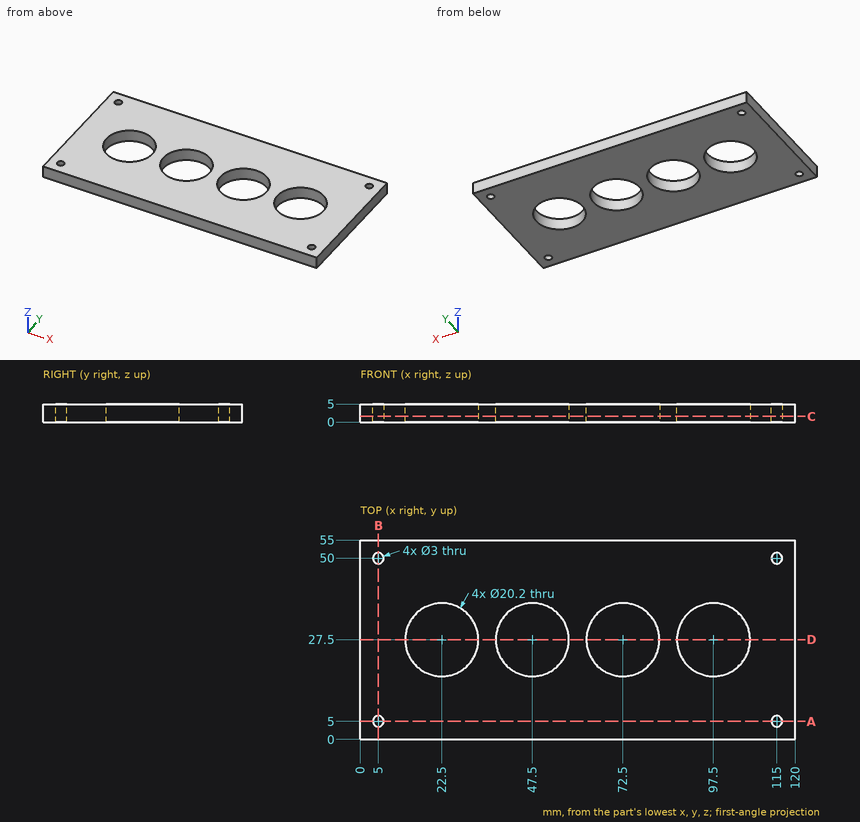
Print and shaded views of the part. All mm, measured from the part's lowest x, y and z. Give positions to 0.01 mm unless a question says otherwise; leave off trailing zeros. Write each loop counter-clockwise with the first axis right and the second up, starting at its lowest first coordinate (ties: lowest second). Pieces come first, ordered by that corner, then holes. Notation, with made-up numbers: (-32.75, 86.25) -> (5.25, 86.25) arc R26 cw to (5.25, 106.25) -> close; hole circle Ø11 at (-23.75, 88). An arc over 180 degrees is marked (long way). Write item = value, one per line.
(1) Slice it at A-A, the plane y = 5. Give the cut face in (x, z), then the cut area to 3 significant figures.
Determined:
outline = (0, 0) -> (3.5, 0) -> (3.5, 5) -> (0, 5) -> close; (6.5, 0) -> (113.5, 0) -> (113.5, 5) -> (6.5, 5) -> close; (116.5, 0) -> (120, 0) -> (120, 5) -> (116.5, 5) -> close
area = 570 mm2
(2) Slice it at C-C, the plane z = 1.6. Give the number of separate pieces and of enclosed holes in the cut face, then the cut area to 3 significant figures.
Determined:
separate_pieces = 1
enclosed_holes = 8
area = 5,290 mm2
(3) Probe line 1 along X through (y, z) = (22.5, 3); line 2 along X through (y, z) = (19, 2.05); line 3 along Y through (x, z) = (72.5, 2.7). List the from-to ranges inside material, lowest first.
Determined:
line_1 = 0 to 13.72, 31.28 to 38.72, 56.28 to 63.72, 81.28 to 88.72, 106.28 to 120
line_2 = 0 to 17.04, 27.96 to 42.04, 52.96 to 67.04, 77.96 to 92.04, 102.96 to 120
line_3 = 0 to 17.4, 37.6 to 55
(4) Slice it at B-B, the plane x = 5. Give the cut face in (y, z), then the cut area to 3 significant figures.
Determined:
outline = (0, 0) -> (3.5, 0) -> (3.5, 5) -> (0, 5) -> close; (6.5, 0) -> (48.5, 0) -> (48.5, 5) -> (6.5, 5) -> close; (51.5, 0) -> (55, 0) -> (55, 5) -> (51.5, 5) -> close
area = 245 mm2
(5) Slice it at D-D, the plane y = 27.5. Give the cut face in (x, z), then the cut area to 3 significant figures.
Determined:
outline = (0, 0) -> (12.4, 0) -> (12.4, 5) -> (0, 5) -> close; (32.6, 0) -> (37.4, 0) -> (37.4, 5) -> (32.6, 5) -> close; (57.6, 0) -> (62.4, 0) -> (62.4, 5) -> (57.6, 5) -> close; (82.6, 0) -> (87.4, 0) -> (87.4, 5) -> (82.6, 5) -> close; (107.6, 0) -> (120, 0) -> (120, 5) -> (107.6, 5) -> close
area = 196 mm2
